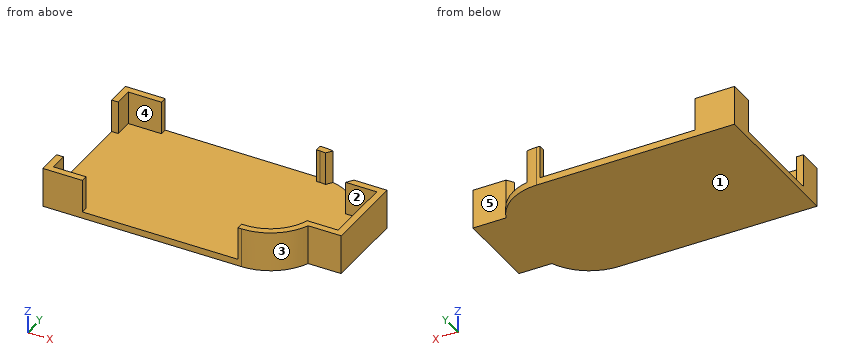
from build123d import *

# Parameters (mm, degrees)
F1_DEPTH  = 2
F3_DEPTH  = 10
F4_W      = 30
F4_H      = 10
F5_DEPTH  = 1.9956371739
F4_H_2    = 50
F6_DEPTH  = 25
F8_DEPTH  = 50
F9_W      = 47
F9_H      = 10
F10_DEPTH = 45.0007863305
F11_SCALE = 1.06


with BuildPart() as f1:
    # F0 (on Top) → F1 (new body)
    with BuildSketch(Plane.XY):
        with BuildLine():
            Line((60, 22.5), (0, 22.5))
            Line((0, 22.5), (0.09805652, -22.4997863305))
            Line((0.09805652, -22.4997863305), (60.0974867347, -22.2383022772))
            ThreePointArc((60.0974867347, -22.2383022772), (68.9331965187, -19.52097203), (74.7776478239, -12.3588466471))
            Line((74.7776478239, -12.3588466471), (84.7775528597, -12.3152659716))
            Line((84.7775528597, -12.3152659716), (84.7230770152, 12.6846153232))
            Line((84.7230770152, 12.6846153232), (74.7230770152, 12.6846153232))
            ThreePointArc((74.7230770152, 12.6846153232), (68.8474681852, 19.8212021779), (60, 22.5))
        make_face()
    extrude(amount=F1_DEPTH)

    # F2 (on face) → F3 (join)
    with BuildSketch(Plane.XY.offset(2)):
        with BuildLine():
            Line((0.09805652, -22.4997863305), (60.0974867347, -22.2383022772))
            ThreePointArc((60.0974867347, -22.2383022772), (68.9331965187, -19.52097203), (74.7776478239, -12.3588466471))
            Line((74.7776478239, -12.3588466471), (84.7775528597, -12.3152659716))
            Line((84.7775528597, -12.3152659716), (84.7230770152, 12.6846153232))
            Line((84.7230770152, 12.6846153232), (74.7230770152, 12.6846153232))
            ThreePointArc((74.7230770152, 12.6846153232), (68.8474681852, 19.8212021779), (60, 22.5))
            Line((60, 22.5), (0, 22.5))
            Line((0, 22.5), (0.09805652, -22.4997863305))
        make_face()
        with BuildLine():
            Line((2, 20.5), (60, 20.5))
            ThreePointArc((60, 20.5), (68.2741953452, 17.7812150693), (73.3231924886, 10.6846153232))
            Line((73.3231924886, 10.6846153232), (82.7230770152, 10.6846153232))
            Line((82.7230770152, 10.6846153232), (82.7230770152, 0.1802572349))
            Line((82.7230770152, 0.1802572349), (82.7688557174, -10.3240010995))
            Line((82.7688557174, -10.3240010995), (73.3690604561, -10.3649664313))
            ThreePointArc((73.3690604561, -10.3649664313), (68.3510387212, -17.4835026557), (60.0887705996, -20.23832127))
            Line((60.0887705996, -20.23832127), (2.0893213921, -20.4910891882))
            Line((2.0893213921, -20.4910891882), (2, 20.5))
        make_face(mode=Mode.SUBTRACT)
    extrude(amount=F3_DEPTH)

    # F4 (on face) → F5 (cut, through all)
    with BuildSketch(Plane(origin=(0.04902826, 0.0001068347, 0), x_dir=(0.002179039, -0.9999976259, 0), z_dir=(-0.9999976259, -0.002179039, 0))):
        with Locations((0, 7)):
            Rectangle(F4_W, F4_H)
    extrude(amount=-F5_DEPTH, mode=Mode.SUBTRACT)

    # F4 (on face) → F6 (cut)
    with BuildSketch(Plane(origin=(0.04902826, 0.0001068347, 0), x_dir=(0.002179039, -0.9999976259, 0), z_dir=(-0.9999976259, -0.002179039, 0))):
        with Locations((0, 27)):
            Rectangle(F4_W, F4_H_2)
    extrude(amount=-F6_DEPTH, mode=Mode.SUBTRACT)

    # F7 (on face) → F8 (cut)
    with BuildSketch(Plane.XY.offset(2)):
        Polygon((56.9224528048, 13.4114075262), (69.6910599869, 5.4954265969), (86.4650020105, 29.460177553), (73.6963948284, 37.3761584823), align=None)
    extrude(amount=F8_DEPTH, mode=Mode.SUBTRACT)

    # F9 (on face) → F10 (cut, through all)
    with BuildSketch(Plane(origin=(0, 22.5, 0), x_dir=(-1, 0, 0), z_dir=(0, 1, 0))):
        with Locations((-35.5, 7)):
            Rectangle(F9_W, F9_H)
    extrude(amount=-F10_DEPTH, mode=Mode.SUBTRACT)


with BuildPart() as f1_1:
    # F11: moved
    add(f1.part.scale(F11_SCALE))


solid = f1_1.part
The model under review builds one solid part; all positions refer to its coordinate system, in mm. Face numbers are marked on the shaded views. A direction names the side the tool comes from. Round coordinates to 2 decimals unless told otherwise and drop trailing zeros. Loops run counter-clockwise (first coordinate to the right, second up) from the corner with the lowest first, then second, coordinate; pieces in that order, holes last. Notation, with made-up numbers: (-33.75, 79.25) -> (-26.75, 79.25) arc R22 cw to (-26.75, 113.25) -> close; hole circle Ø6 at (64.25, 58.25). An arc over 180 degrees is marked (long way). One line per question, with ' | ' between items. Start each with the question number.
Item 1: Machinability: for the marked faces 1 and 2, which of the approach directions +Z, -Z, +X, -X, +Y, -Y give a long, thin tool a straight path to every point of the face, cutting with its end or side? Answer none if there is none.
Item 2: Wall thickness on line 1 along Y through (x, z) = (4.5, 4); line 2 along X through (y, z) = (6.5, 3); line 3 along Z through (x, y) = (63.5, 18): over which ranges is each line inside the solid? List them lowest first. Write a range as [from, to].
Item 3: Add section C-C, the plane x = 83. Write out the cut boundary in (y, z).
Item 4: Add section D-D, the plane y = 6. Write out the cut boundary in (x, z), then the cut area to 3 significant figures.
Item 5: Add section B-B, the plane y = -9.5. Write out the cut boundary in (x, z), then the cut area to 3 significant figures.
Item 6: Add section A-A, the plane z = 4.25. Count the separate pieces of the cut face and the enclosed holes in it, then the cut area to 3 significant figures.
Item 7: Draft analysis for pull direction X (two halves, no side actions). For the marked faces 3, 4 and 5, state which applies: +X half, -X half, draft (parallel to the pull), parting line (faces both ways), or undercut.
Item 8: For pin 1 (5 mm diameter, centred on x = 81.5, z = 8.5, fed in from -Y); pin 2 (2 mm diameter, centred on y = 13, z = 2, fed in from +X); pin 3 (6 mm diameter, centred on y = -19, z = 9, fed in from +X), all flat-tipped, find the tip position at first contact; note any pin that passes through.
Return value:
1) face 1: -Z, +X, -X, +Y, -Y | face 2: +Z, -X
2) line 1: y = [-23.83, -21.71], [21.73, 23.85] | line 2: x = [87.69, 89.82] | line 3: z = [0, 2.12]
3) outline: (-13.08, 0) -> (13.45, 0) -> (13.45, 12.72) -> (11.33, 12.72) -> (11.33, 2.12) -> (-10.96, 2.12) -> (-10.96, 12.72) -> (-13.08, 12.72) -> close
4) outline: (0.04, 0) -> (89.82, 0) -> (89.82, 12.72) -> (87.69, 12.72) -> (87.69, 2.12) -> (0.04, 2.12) -> close | area: 213 mm2
5) outline: (0.07, 0) -> (89.86, 0) -> (89.86, 12.72) -> (87.73, 12.72) -> (87.73, 2.12) -> (0.07, 2.12) -> close | area: 213 mm2
6) separate pieces: 4 | enclosed holes: 0 | area: 225 mm2
7) face 3: +X half | face 4: undercut | face 5: draft
8) pin 1: stops at y = -13.71 | pin 2: stops at x = 89.81 | pin 3: stops at x = 77.73
